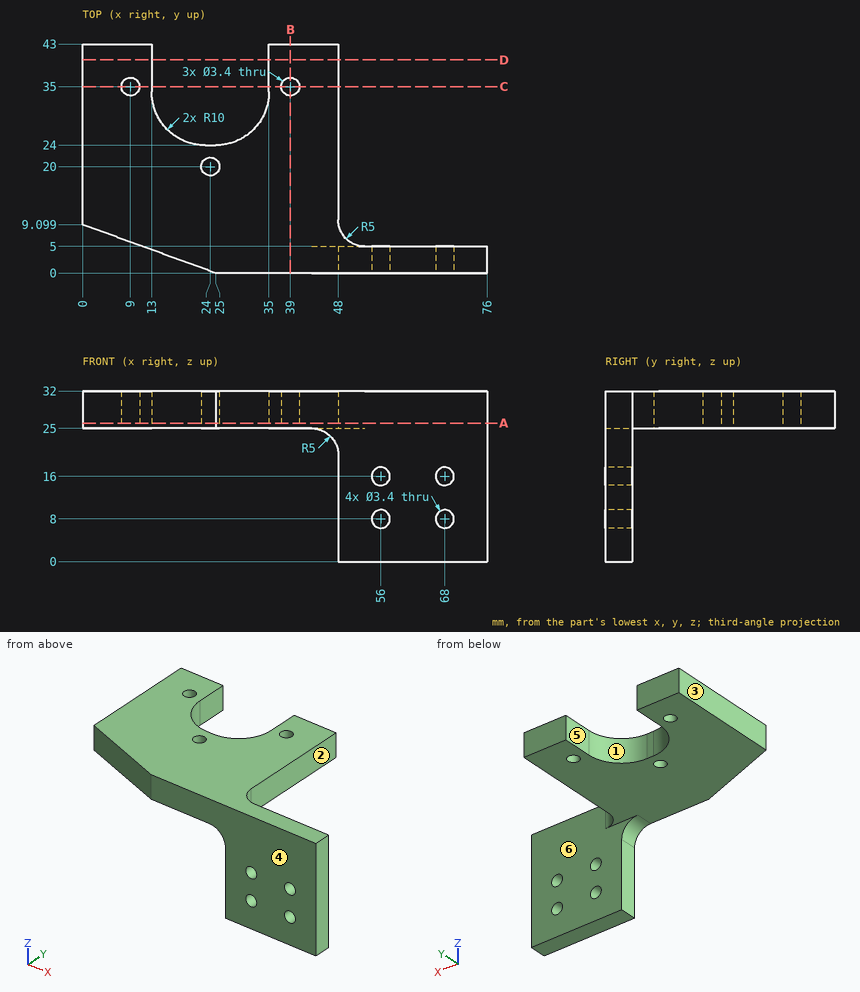
Geometry: see drawing. Coordinates: mm, zero at the bounding-box minimum. A direction names the side the tool comes from. Round coordinates to 2 decimals unless told otherwise and drop trailing zeros. Write each loop counter-clockwise with the first axis right and the second up, starting at its lowest first coordinate (ties: lowest second). Pieces come first, ordered by that corner, then holes. Notation, with made-up numbers: (27, 77) -> (62, 77) arc R8 cw to (62, 87) -> close; hole circle Ø7 at (-38.75, 5). An arc over 180 degrees is marked (long way). Answer as CSV lines item,"result".
1. Section A-A (z = 26). Return the cut outline in (x, y).
Geometry says:
outline,"(0, 9.1) -> (25, 0) -> (76, 0) -> (76, 5) -> (53, 5) arc R5 cw to (48, 10) -> (48, 43) -> (35, 43) -> (35, 34) arc R10 cw to (25, 24) -> (23, 24) arc R10 cw to (13, 34) -> (13, 43) -> (0, 43) -> close; hole circle Ø3.4 at (9, 35); hole circle Ø3.4 at (24, 20); hole circle Ø3.4 at (39, 35)"
2. Contact query for flat-ended pins moving along their axis: P1, Ø5.5, axis at x = 56, z = 8, coming from the +Y side; P2, Ø5.5, axis at y = 25, z = 27, coming from the +X side; P3, Ø8, axis at x = 13, y = 8, coming from the -Z side. Output: stop coordinate, or through.
Geometry says:
P1,"stops at y = 5"
P2,"stops at x = 48"
P3,"stops at z = 25"
3. Reachability of the marked faces 4, 5 and 6 from +Z, -Z, +X, -X, +Y, -Y: full face, straight path, thin tool, end or side. Return the list, or none.
Geometry says:
face 4,"+Z, -Z, +X, -X, -Y"
face 5,"+Z, -Z, +Y"
face 6,"-Z, +X, +Y"
4. Section D-D (y = 40). Return the cut outline in (x, z).
Geometry says:
outline,"(0, 25) -> (13, 25) -> (13, 32) -> (0, 32) -> close; (35, 25) -> (48, 25) -> (48, 32) -> (35, 32) -> close"
5. Mould query, pull axis X, two halves, no side actions, for the marked faces 1, 2 and 3. Classes: +X half, -X half, draft (parallel to the pull), parting line (faces both ways), or undercut.
Geometry says:
face 1,"undercut"
face 2,"+X half"
face 3,"-X half"
6. Section B-B (x = 39). Return the cut outline in (y, z).
Geometry says:
outline,"(0, 25) -> (33.3, 25) -> (33.3, 32) -> (0, 32) -> close; (36.7, 25) -> (43, 25) -> (43, 32) -> (36.7, 32) -> close"
7. Ray query, L1, parallel to Z at x = 56, y = 1; L2, parallel to X at y = 1.6, z = 8; L3, parallel to X at y = 41, z = 29. Return the intervals inside material, ascending. Write a range as [from, to].
Geometry says:
L1,"z = [0, 6.3], [9.7, 14.3], [17.7, 32]"
L2,"x = [48, 54.3], [57.7, 66.3], [69.7, 76]"
L3,"x = [0, 13], [35, 48]"
8. Section C-C (y = 35). Return the cut outline in (x, z).
Geometry says:
outline,"(0, 25) -> (7.3, 25) -> (7.3, 32) -> (0, 32) -> close; (10.7, 25) -> (13, 25) -> (13, 32) -> (10.7, 32) -> close; (35, 25) -> (37.3, 25) -> (37.3, 32) -> (35, 32) -> close; (40.7, 25) -> (48, 25) -> (48, 32) -> (40.7, 32) -> close"
